Input: part model. Units: mm. Frame: model coordinates. A direction names the side the tool comes from. Give positions to 0.01 mm unless a question says otherwise; leave off trailing zeros. Order: outer loops, then holes, each group sorted by start corner. A loop starts at its lowest first (then second) coordinate and runs counter-clockwise, first axis right, second up. Notation, with made-up numbers: (31, 14) - (42, 14) arc R26 ccw to (42, 44) - close; hole circle Ø1 at (-38.5, -5). An arc over 180 degrees is marked (long way). Use a Markdown table: item, result.
from build123d import *

# Parameters (mm, degrees)
F0_W     = 1
F0_H     = 15
F0_W_2   = 15
F0_H_2   = 1
F1_DEPTH = 1
F2_DEPTH = 16
F3_W     = 2
F3_H     = 3
F3_W_2   = 3
F3_H_2   = 2
F4_DEPTH = 3
F5_W     = 1
F5_H     = 1
F6_DEPTH = 25
F7_DEPTH = 15
F9_DEPTH = 1


with BuildPart() as f1:
    # F0 (on Top) → F1 (new body)
    with BuildSketch(Plane.XY):
        with Locations((8, 0)):
            Rectangle(F0_W, F0_H)
        with Locations((-16, -8)):
            Rectangle(F0_W_2, F0_H_2)
        with Locations((-16, 0)):
            Rectangle(F0_W_2, F0_H)
        with Locations((8, -16)):
            Rectangle(F0_W, F0_H)
        with Locations((0, -16)):
            Rectangle(F0_W_2, F0_H)
        with Locations((-8, -16)):
            Rectangle(F0_W, F0_H)
        with Locations((16, -16)):
            Rectangle(F0_W_2, F0_H)
        with Locations((-16, -16)):
            Rectangle(F0_W_2, F0_H)
        with Locations((16, 0)):
            Rectangle(F0_W_2, F0_H)
        with Locations((16, -8)):
            Rectangle(F0_W_2, F0_H_2)
        with Locations((0, -8)):
            Rectangle(F0_W_2, F0_H_2)
        with Locations((-8, 0)):
            Rectangle(F0_W, F0_H)
        Rectangle(F0_W_2, F0_H)
        with Locations((8, -8)):
            Rectangle(F0_W, F0_H_2)
        with Locations((-8, -8)):
            Rectangle(F0_W, F0_H_2)
        with Locations((-8, 8)):
            Rectangle(F0_W, F0_H_2)
        with Locations((-16, 8)):
            Rectangle(F0_W_2, F0_H_2)
        with Locations((8, 16)):
            Rectangle(F0_W, F0_H)
        with Locations((0, 16)):
            Rectangle(F0_W_2, F0_H)
        with Locations((-8, 16)):
            Rectangle(F0_W, F0_H)
        with Locations((16, 16)):
            Rectangle(F0_W_2, F0_H)
        with Locations((16, 8)):
            Rectangle(F0_W_2, F0_H_2)
        with Locations((-16, 16)):
            Rectangle(F0_W_2, F0_H)
        with Locations((8, 8)):
            Rectangle(F0_W, F0_H_2)
        with Locations((0, 8)):
            Rectangle(F0_W_2, F0_H_2)
    extrude(amount=-F1_DEPTH)

    # F0 (on Top) → F2 (join)
    with BuildSketch(Plane.XY):
        with Locations((-8, -8)):
            Rectangle(F0_W, F0_H_2)
        with Locations((8, -8)):
            Rectangle(F0_W, F0_H_2)
        with Locations((-8, 8)):
            Rectangle(F0_W, F0_H_2)
        with Locations((8, 8)):
            Rectangle(F0_W, F0_H_2)
        with Locations((16, 8)):
            Rectangle(F0_W_2, F0_H_2)
        with Locations((8, 16)):
            Rectangle(F0_W, F0_H)
        with Locations((-8, 16)):
            Rectangle(F0_W, F0_H)
        with Locations((0, 8)):
            Rectangle(F0_W_2, F0_H_2)
        with Locations((-16, 8)):
            Rectangle(F0_W_2, F0_H_2)
        with Locations((-8, 0)):
            Rectangle(F0_W, F0_H)
        with Locations((-16, -8)):
            Rectangle(F0_W_2, F0_H_2)
        with Locations((0, -8)):
            Rectangle(F0_W_2, F0_H_2)
        with Locations((16, -8)):
            Rectangle(F0_W_2, F0_H_2)
        with Locations((8, -16)):
            Rectangle(F0_W, F0_H)
        with Locations((-8, -16)):
            Rectangle(F0_W, F0_H)
        with Locations((8, 0)):
            Rectangle(F0_W, F0_H)
    extrude(amount=F2_DEPTH)

    # F3 (on face) → F4 (cut)
    with BuildSketch(Plane(origin=(0, 0, -1), x_dir=(1, 0, 0), z_dir=(0, 0, -1))):
        with BuildLine():
            Line((-7.5, 8.25), (-7.5, 7.5))
            Line((-7.5, 7.5), (-6.75, 7.5))
            ThreePointArc((-6.75, 7.5), (-6.9696699141, 8.0303300859), (-7.5, 8.25))
        make_face()
        with BuildLine():
            Line((-6.75, 7.5), (-7.5, 7.5))
            Line((-7.5, 7.5), (-7.5, 6.75))
            ThreePointArc((-7.5, 6.75), (-6.9696699141, 6.9696699141), (-6.75, 7.5))
        make_face()
        with BuildLine():
            Line((-7.5, 6.75), (-7.5, 7.5))
            Line((-7.5, 7.5), (-8.25, 7.5))
            ThreePointArc((-8.25, 7.5), (-8.0303300859, 6.9696699141), (-7.5, 6.75))
        make_face()
        with BuildLine():
            Line((-8.25, 7.5), (-7.5, 7.5))
            Line((-7.5, 7.5), (-7.5, 8.25))
            ThreePointArc((-7.5, 8.25), (-8.0303300859, 8.0303300859), (-8.25, 7.5))
        make_face()
        with BuildLine():
            Line((-1, 7.5), (-6.75, 7.5))
            ThreePointArc((-6.75, 7.5), (-6.9696699141, 6.9696699141), (-7.5, 6.75))
            Line((-7.5, 6.75), (-7.5, 1))
            Line((-7.5, 1), (-7.5, -1))
            Line((-7.5, -1), (-7.5, -6.75))
            ThreePointArc((-7.5, -6.75), (-6.9696699141, -6.9696699141), (-6.75, -7.5))
            Line((-6.75, -7.5), (-1, -7.5))
            Line((-1, -7.5), (1, -7.5))
            Line((1, -7.5), (6.75, -7.5))
            ThreePointArc((6.75, -7.5), (6.9696699141, -6.9696699141), (7.5, -6.75))
            Line((7.5, -6.75), (7.5, -1))
            Line((7.5, -1), (7.5, 1))
            Line((7.5, 1), (7.5, 6.75))
            ThreePointArc((7.5, 6.75), (6.9696699141, 6.9696699141), (6.75, 7.5))
            Line((6.75, 7.5), (1, 7.5))
            Line((1, 7.5), (-1, 7.5))
        make_face()
        with BuildLine():
            Line((-10.5, 7.5), (-8.25, 7.5))
            ThreePointArc((-8.25, 7.5), (-8.0303300859, 8.0303300859), (-7.5, 8.25))
            Line((-7.5, 8.25), (-7.5, 10.5))
            Line((-7.5, 10.5), (-10.5, 10.5))
            Line((-10.5, 10.5), (-10.5, 7.5))
        make_face()
        with Locations((0, 9)):
            Rectangle(F3_W, F3_H)
        with Locations((-9, 0)):
            Rectangle(F3_W_2, F3_H_2)
        with BuildLine():
            ThreePointArc((7.5, 8.25), (6.9696699141, 8.0303300859), (6.75, 7.5))
            Line((6.75, 7.5), (7.5, 7.5))
            Line((7.5, 7.5), (7.5, 8.25))
        make_face()
        with BuildLine():
            Line((7.5, 7.5), (6.75, 7.5))
            ThreePointArc((6.75, 7.5), (6.9696699141, 6.9696699141), (7.5, 6.75))
            Line((7.5, 6.75), (7.5, 7.5))
        make_face()
        with BuildLine():
            ThreePointArc((-6.75, -7.5), (-6.9696699141, -6.9696699141), (-7.5, -6.75))
            Line((-7.5, -6.75), (-7.5, -7.5))
            Line((-7.5, -7.5), (-6.75, -7.5))
        make_face()
        with BuildLine():
            Line((-7.5, -7.5), (-7.5, -6.75))
            ThreePointArc((-7.5, -6.75), (-8.0303300859, -6.9696699141), (-8.25, -7.5))
            Line((-8.25, -7.5), (-7.5, -7.5))
        make_face()
        with BuildLine():
            Line((8.25, 7.5), (7.5, 7.5))
            Line((7.5, 7.5), (7.5, 6.75))
            ThreePointArc((7.5, 6.75), (8.0303300859, 6.9696699141), (8.25, 7.5))
        make_face()
        with BuildLine():
            Line((7.5, 8.25), (7.5, 7.5))
            Line((7.5, 7.5), (8.25, 7.5))
            ThreePointArc((8.25, 7.5), (8.0303300859, 8.0303300859), (7.5, 8.25))
        make_face()
        with BuildLine():
            Line((7.5, 10.5), (7.5, 8.25))
            ThreePointArc((7.5, 8.25), (8.0303300859, 8.0303300859), (8.25, 7.5))
            Line((8.25, 7.5), (10.5, 7.5))
            Line((10.5, 7.5), (10.5, 10.5))
            Line((10.5, 10.5), (7.5, 10.5))
        make_face()
        with BuildLine():
            Line((-7.5, -8.25), (-7.5, -7.5))
            Line((-7.5, -7.5), (-8.25, -7.5))
            ThreePointArc((-8.25, -7.5), (-8.0303300859, -8.0303300859), (-7.5, -8.25))
        make_face()
        with BuildLine():
            Line((-6.75, -7.5), (-7.5, -7.5))
            Line((-7.5, -7.5), (-7.5, -8.25))
            ThreePointArc((-7.5, -8.25), (-6.9696699141, -8.0303300859), (-6.75, -7.5))
        make_face()
        with BuildLine():
            ThreePointArc((-7.5, -8.25), (-8.0303300859, -8.0303300859), (-8.25, -7.5))
            Line((-8.25, -7.5), (-10.5, -7.5))
            Line((-10.5, -7.5), (-10.5, -10.5))
            Line((-10.5, -10.5), (-7.5, -10.5))
            Line((-7.5, -10.5), (-7.5, -8.25))
        make_face()
        with Locations((9, 0)):
            Rectangle(F3_W_2, F3_H_2)
        with Locations((0, -9)):
            Rectangle(F3_W, F3_H)
        with BuildLine():
            ThreePointArc((8.25, -7.5), (8.0303300859, -6.9696699141), (7.5, -6.75))
            Line((7.5, -6.75), (7.5, -7.5))
            Line((7.5, -7.5), (8.25, -7.5))
        make_face()
        with BuildLine():
            Line((7.5, -7.5), (7.5, -6.75))
            ThreePointArc((7.5, -6.75), (6.9696699141, -6.9696699141), (6.75, -7.5))
            Line((6.75, -7.5), (7.5, -7.5))
        make_face()
        with BuildLine():
            Line((7.5, -7.5), (6.75, -7.5))
            ThreePointArc((6.75, -7.5), (6.9696699141, -8.0303300859), (7.5, -8.25))
            Line((7.5, -8.25), (7.5, -7.5))
        make_face()
        with BuildLine():
            Line((8.25, -7.5), (7.5, -7.5))
            Line((7.5, -7.5), (7.5, -8.25))
            ThreePointArc((7.5, -8.25), (8.0303300859, -8.0303300859), (8.25, -7.5))
        make_face()
        with BuildLine():
            Line((10.5, -7.5), (8.25, -7.5))
            ThreePointArc((8.25, -7.5), (8.0303300859, -8.0303300859), (7.5, -8.25))
            Line((7.5, -8.25), (7.5, -10.5))
            Line((7.5, -10.5), (10.5, -10.5))
            Line((10.5, -10.5), (10.5, -7.5))
        make_face()
    extrude(amount=-F4_DEPTH, mode=Mode.SUBTRACT)

    # F5 (on face) → F6 (cut)
    with BuildSketch(Plane.XY.offset(16)):
        with Locations((-8, 23)):
            Rectangle(F5_W, F5_H)
        with Locations((-23, 8)):
            Rectangle(F5_W, F5_H)
        with Locations((8, 23)):
            Rectangle(F5_W, F5_H)
        with Locations((23, 8)):
            Rectangle(F5_W, F5_H)
        with Locations((23, -8)):
            Rectangle(F5_W, F5_H)
        with Locations((8, -23)):
            Rectangle(F5_W, F5_H)
        with Locations((-8, -23)):
            Rectangle(F5_W, F5_H)
        with Locations((-23, -8)):
            Rectangle(F5_W, F5_H)
    extrude(amount=-F6_DEPTH, mode=Mode.SUBTRACT)

    # F5 (on face) → F7 (join)
    with BuildSketch(Plane.XY.offset(16)):
        with Locations((-8, 23)):
            Rectangle(F5_W, F5_H)
        with Locations((-23, 8)):
            Rectangle(F5_W, F5_H)
        with Locations((8, 23)):
            Rectangle(F5_W, F5_H)
        with Locations((23, 8)):
            Rectangle(F5_W, F5_H)
        with Locations((23, -8)):
            Rectangle(F5_W, F5_H)
        with Locations((8, -23)):
            Rectangle(F5_W, F5_H)
        with Locations((-8, -23)):
            Rectangle(F5_W, F5_H)
        with Locations((-23, -8)):
            Rectangle(F5_W, F5_H)
    extrude(amount=-F7_DEPTH)

    # F8 (on Top) → F9 (join)
    with BuildSketch(Plane.XY):
        Polygon((-1, 7.5), (-5.5, 7.5), (-5.5, 5.5), (-7.5, 5.5), (-7.5, 1), (-6.5, 1), (-6.5, -1), (-7.5, -1), (-7.5, -5.5), (-5.5, -5.5), (-5.5, -7.5), (-1, -7.5), (-1, -5.5), (1, -5.5), (1, -7.5), (5.5, -7.5), (5.5, -5.5), (7.5, -5.5), (7.5, -1), (5.5, -1), (5.5, 1), (7.5, 1), (7.5, 5.5), (5.5, 5.5), (5.5, 7.5), (1, 7.5), (1, 5.5), (-1, 5.5), align=None)
    extrude(amount=F9_DEPTH)


solid = f1.part
1. Mould query, pull axis Y, two halves, no side actions, for faces 6 (the face through (9.1, 7.5, -0.2)), 7 (the face through (-16, 16, 0)), 8 (the face through (16, -8.5, 8)). Classes: pulls with the +Y half, pulls with the -Y half, needs draft (parallel to the pull), parting line crosses it, or undercut.
Response:
| item | result |
|---|---|
| face 6 | undercut |
| face 7 | needs draft |
| face 8 | pulls with the -Y half |
2. Section query A-A (y = 14). Return loops of the section in (x, z).
Response:
| item | result |
|---|---|
| outline | (-23.5, -1) - (23.5, -1) - (23.5, 0) - (8.5, 0) - (8.5, 16) - (7.5, 16) - (7.5, 0) - (-7.5, 0) - (-7.5, 16) - (-8.5, 16) - (-8.5, 0) - (-23.5, 0) - close |
3. Pin query (flat end, axial travel): pin 1 (4.5 mm diameter, centred on x = 16, y = -3, fed in from +Z); pin 2 (2 mm diameter, centred on x = -7, z = 9.5, fed in from +Y); pin 3 (0.5 mm diameter, centred on y = -8, z = 0, fed in from -X); pin 4 (4.5 mm diameter, centred on x = -1.5, z = 8, fed in from +Y). Return the tip coordinate at first contact, or that it passes through.
Response:
| item | result |
|---|---|
| pin 1 | stops at z = 0 |
| pin 2 | stops at y = 23.5 |
| pin 3 | stops at x = -22.5 |
| pin 4 | stops at y = 8.5 |
4. Set-up query: faces 1 (the face through (8, -8, 2)), 2 (the face through (0, 8.5, 8)), 3 (the face through (8.5, -16, 8)), 4 (the face through (8.5, 16, 8)), 5 (the face through (-11, 0, -1)). Return all of +Z, -Z, +X, -X, +Y, -Y with unobstructed straight access to the full face (end or side cutting, diameter ignored); none if empty.
Response:
| item | result |
|---|---|
| face 1 | -Z |
| face 2 | +Z, +Y |
| face 3 | +Z, +X, -Y |
| face 4 | +Z, +X, +Y |
| face 5 | -Z, +X, -X, +Y, -Y |
5. Material intervals for line 1 along X through (y, z) = (-1, 6.5); line 2 along Z through (x, y) = (20, 2), sorted ascending.
Response:
| item | result |
|---|---|
| line 1 | x = -8.5 to -7.5, 7.5 to 8.5 |
| line 2 | z = -1 to 0 |
